Autodesk Inventor part; units mm, degrees
ref_plane "YZ Plane" through (0, 0, 0) normal (1, 0, 0) x (0, 1, 0)
ref_plane "XZ Plane" through (0, 0, 0) normal (0, 1, 0) x (-1, 0, 0)
ref_plane "XY Plane" through (0, 0, 0) normal (0, 0, 1) x (1, 0, 0)
sketch "Boceto1" plane through (0, 0, 0) normal (0, 0, 1) x (1, 0, 0)
  line L0 (0, 0) -> (0, 210)
  line L1 (0, 210) -> (450, 210)
  line L2 (450, 210) -> (450, 0)
  line L3 (450, 0) -> (0, 0)
  line L4 (5, 5) -> (50, 5)
  line L5 (50, 5) -> (50, 8)
  line L6 (5, 5) -> (5, 35.71)
  line L7 (5, 35.71) -> (8, 35.71)
  line L8 (50, 8) -> (8, 8)
  line L9 (8, 8) -> (8, 35.71)
  line L10 (5, 63.43) -> (5, 91.14)
  line L11 (5, 118.86) -> (5, 146.57)
  line L12 (5, 174.29) -> (5, 205)
  line L13 (5, 63.43) -> (8, 63.43)
  line L14 (8, 63.43) -> (8, 91.14)
  line L15 (8, 91.14) -> (5, 91.14)
  line L16 (5, 118.86) -> (8, 118.86)
  line L17 (8, 118.86) -> (8, 146.57)
  line L18 (8, 146.57) -> (5, 146.57)
  line L19 (5, 205) -> (50, 205)
  line L20 (50, 205) -> (50, 202)
  line L21 (50, 202) -> (8, 202)
  line L22 (8, 202) -> (8, 174.29)
  line L23 (8, 174.29) -> (5, 174.29)
  line L24 (100, 205) -> (150, 205)
  line L25 (200, 205) -> (250, 205)
  line L26 (300, 205) -> (350, 205)
  line L27 (400, 205) -> (445, 205)
  line L28 (100, 205) -> (100, 202)
  line L29 (100, 202) -> (150, 202)
  line L30 (150, 202) -> (150, 205)
  line L31 (200, 205) -> (200, 202)
  line L32 (200, 202) -> (250, 202)
  line L33 (250, 202) -> (250, 205)
  line L34 (300, 205) -> (300, 202)
  line L35 (300, 202) -> (350, 202)
  line L36 (350, 202) -> (350, 205)
  line L37 (445, 205) -> (445, 174.29)
  line L38 (400, 205) -> (400, 202)
  line L39 (400, 202) -> (442, 202)
  line L40 (442, 202) -> (442, 174.29)
  line L41 (442, 174.29) -> (445, 174.29)
  line L42 (100, 5) -> (150, 5)
  line L43 (200, 5) -> (250, 5)
  line L44 (300, 5) -> (350, 5)
  line L45 (400, 5) -> (445, 5)
  line L46 (100, 5) -> (100, 8)
  line L47 (100, 8) -> (150, 8)
  line L48 (150, 8) -> (150, 5)
  line L49 (200, 5) -> (200, 8)
  line L50 (200, 8) -> (250, 8)
  line L51 (250, 8) -> (250, 5)
  line L52 (300, 5) -> (300, 8)
  line L53 (300, 8) -> (350, 8)
  line L54 (350, 8) -> (350, 5)
  line L55 (445, 5) -> (445, 35.71)
  line L56 (445, 35.71) -> (442, 35.71)
  line L57 (400, 5) -> (400, 8)
  line L58 (400, 8) -> (442, 8)
  line L59 (442, 8) -> (442, 35.71)
  line L60 (445, 63.43) -> (445, 91.14)
  line L61 (445, 118.86) -> (445, 146.57)
  line L62 (445, 63.43) -> (442, 63.43)
  line L63 (442, 63.43) -> (442, 91.14)
  line L64 (442, 91.14) -> (445, 91.14)
  line L65 (445, 118.86) -> (442, 118.86)
  line L66 (442, 118.86) -> (442, 146.57)
  line L67 (442, 146.57) -> (445, 146.57)
  dimension "d0" = 210
  dimension "d1" = 450
  dimension "d2" = 210
  dimension "d3" = 45
  dimension "d4" = 3
  dimension "d5" = 30.71
  dimension "d7" = 42
  dimension "d8" = 3
  dimension "d9" = 27.72
  dimension "d10" = 27.71
  dimension "d11" = 27.72
  dimension "d12" = 27.71
  dimension "d13" = 27.72
  dimension "d14" = 30.71
  dimension "d15" = 3
  dimension "d16" = 27.71
  dimension "d17" = 3
  dimension "d18" = 27.71
  dimension "d19" = 45
  dimension "d20" = 3
  dimension "d21" = 42
  dimension "d22" = 50
  dimension "d23" = 50
  dimension "d24" = 50
  dimension "d25" = 50
  dimension "d26" = 50
  dimension "d27" = 50
  dimension "d28" = 50
  dimension "d29" = 45
  dimension "d31" = 3
  dimension "d32" = 50
  dimension "d33" = 3
  dimension "d34" = 50
  dimension "d35" = 3
  dimension "d36" = 50
  dimension "d37" = 30.71
  dimension "d38" = 3
  dimension "d39" = 42
  dimension "d40" = 50
  dimension "d41" = 50
  dimension "d42" = 50
  dimension "d43" = 50
  dimension "d44" = 50
  dimension "d45" = 50
  dimension "d46" = 50
  dimension "d47" = 45
  dimension "d51" = 3
  dimension "d52" = 50
  dimension "d53" = 3
  dimension "d54" = 50
  dimension "d55" = 3
  dimension "d56" = 50
  dimension "d57" = 30.71
  dimension "d58" = 3
  dimension "d59" = 3
  dimension "d60" = 27.72
  dimension "d61" = 27.71
  dimension "d62" = 27.72
  dimension "d63" = 27.71
  dimension "d64" = 3
  dimension "d65" = 3
  dimension "d69" = 5
  dimension "d71" = 5
  dimension "d72" = 5
extrude "Extrusión1" add sketch "Boceto1" along normal blind 3
properties part number "Cara frontal 2" material "Madera (cerezo)"
Verification items for the finished model (mm, model axes). Round coordinates to 2 decimals unless told otherwise and drop trailing zeros. Loops run counter-clockwise (first coordinate to the right, second up) from the corner with the lowest first, then second, coordinate; pieces in that order, holes last. Notation, with made-up numbers: (-7, 18) -> (50, 18) arc R30 cw to (50, 51) -> close; hole circle Ø8 at (71, 18). An arc over 180 degrees is marked (long way). Answer as a JSON object with one key per item and string values.
Q1. Section check B-B (z = 0.5). State how many separate pieces and enclosed holes the cut face has, then the cut area to 3 significant figures.
Data:
{"separate pieces": "1", "enclosed holes": "14", "area": "92,400 mm2"}
Q2. Section check A-A (x = 28.5). Record the boundary of the cut face in (y, z), then the cut area to 3 significant figures.
Data:
{"outline": "(0, 0) -> (5, 0) -> (5, 3) -> (0, 3) -> close; (8, 0) -> (202, 0) -> (202, 3) -> (8, 3) -> close; (205, 0) -> (210, 0) -> (210, 3) -> (205, 3) -> close", "area": "612 mm2"}
Q3. Scan lines: line 1 (Y direction, x = 32.5, z = 1.6); line 2 (X direction, y = 145, z = 1.2). Record each from-to range of solid material in increasing order. Write a range as from..to.
Data:
{"line 1": "y = 0..5, 8..202, 205..210", "line 2": "x = 0..5, 8..442, 445..450"}
